Could you check a few things on this model? Use its own coordinates, in mm. Face numbers are marked on the shaded views. A direction names the side the tool comes from. Round coordinates to 2 decimals unless told otherwise and drop trailing zeros. Order: outer loops, then holes, each group sorted by start corner. A loop starts at its lowest first (then second) coordinate and runs counter-clockwise, first axis right, second up. Notation, with made-up numbers: M -23,-38.75 L -11,-38.75 A6 cw -11,-34.75 Z; hole C 41.25,-35 d5. An arc over 180 degrees is marked long. Write each question's results on one line, items separated by ' | '. Start each with the question number.
1. Suppose I cut it at C-C on x = -1. Write out the boundary of the cut face in (y, z), and give its area (4 significant figures).
2. Please list where these lines run through material, in increasing order: L1, parallel to X at y = 40.5, z = 5; L2, parallel to Y at x = 12.5, z = 1.4; L3, parallel to X at y = 30, z = 9.5.
3. Suppose I cut it at A-A on z = 13.5. Write out the boundary of the cut face in (x, y), and give its area (3 significant figures).
4. We'd pull the mould along X, two halves only. Please class the marked faces 1, 2 and 3: released by +X, released by -X, zero draft, split by the parting line, or undercut.
5. Suppose I cut it at B-B on y = 44. Write out the boundary of the cut face in (x, z).
6. I'm going to push flat-ended pins straight in: pin 1 (3 mm diameter, centred on y = 47.5, z = 3, fed in from -X); pin 2 (8 mm diameter, centred on x = 1, z = 5.5, fed in from +Y); pin 3 (1.8 mm diameter, centred on x = 12.5, y = 1.5, fed in from +Z); pin 4 (1.5 mm diameter, centred on x = 22, y = 0, fed in from +Z). Where does each tip first touch, or does it pass through?
7. For the marked faces 4, 5, 6, 7 and 8, which set-ups out of +Z, -Z, +X, -X, +Y, -Y let a thin tool reach every point of the face, with its end or its side?
8. Suppose I cut it at D-D on y = 22.5. Write out the boundary of the cut face in (x, z).
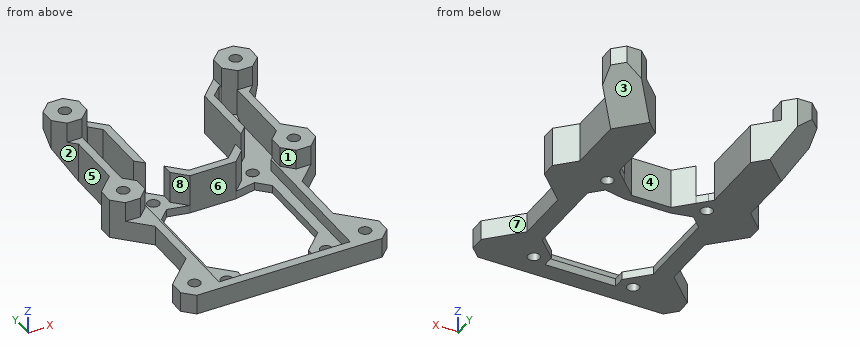
from build123d import *

# Parameters (mm, degrees)
SKETCH5_R           = 1.5
BOSS_EXTRUDE1_DEPTH = 2
SKETCH9_R           = 1.5
BOSS_EXTRUDE3_DEPTH = 3
SKETCH10_R          = 1.5
BOSS_EXTRUDE4_DEPTH = 5
BOSS_EXTRUDE5_DEPTH = 5.1
SKETCH13_R          = 1.5
CUT_EXTRUDE1_DEPTH  = 4.5
CUT_EXTRUDE2_DEPTH  = 7.5
CUT_EXTRUDE3_DEPTH  = 7.5
CHAMFER1_SIZE       = 1
CHAMFER1_SIZE2      = 1.191753593


with BuildPart() as part:
    # Sketch5 → Boss-Extrude1 (new body)
    with BuildSketch(Plane.XY):
        Polygon((19.636038969, -4.5), (-19.636038969, -4.5), (-23.363961031, -4.5), (-26, -1.863961031), (-26, 1.863961031), (-23.363961031, 4.5), (-18.5, 9.363961031), (-18.5, 23.636038969), (-23.363961031, 28.5), (-26, 31.136038969), (-26, 34.863961031), (-23.363961031, 37.5), (-21.5, 39.363961031), (-21.5, 53.636038969), (-23.363961031, 55.5), (-26, 58.136038969), (-26, 61.863961031), (-23.363961031, 64.5), (-19.636038969, 64.5), (-17, 61.863961031), (-12, 56.863961031), (-12, 40.029437252), (-11.050252532, 39.079689783), (-9, 37.029437252), (-4.970562748, 33), (4.970562748, 33), (9, 37.029437252), (11.050252532, 39.079689783), (12, 40.029437252), (12, 56.863961031), (17, 61.863961031), (19.636038969, 64.5), (23.363961031, 64.5), (26, 61.863961031), (26, 58.136038969), (23.363961031, 55.5), (21.5, 53.636038969), (21.5, 39.363961031), (23.363961031, 37.5), (26, 34.863961031), (26, 31.136038969), (23.363961031, 28.5), (18.5, 23.636038969), (18.5, 9.363961031), (23.363961031, 4.5), (26, 1.863961031), (26, -1.863961031), (23.363961031, -4.5), align=None)
        with Locations((-12.5, 35.579689783)):
            Circle(SKETCH5_R, mode=Mode.SUBTRACT)
        with Locations((-12.5, 1.5)):
            Circle(SKETCH5_R, mode=Mode.SUBTRACT)
        with Locations((12.5, 1.5)):
            Circle(SKETCH5_R, mode=Mode.SUBTRACT)
        with Locations((12.5, 35.579689783)):
            Circle(SKETCH5_R, mode=Mode.SUBTRACT)
        Polygon((-5.798989873, 31), (5.798989873, 31), (11.050252532, 32.079689783), (14, 29.129942315), (14, 8.121320344), (11, 5.121320344), (8.878679656, 3), (8.878679656, 0), (-8.878679656, 0), (-8.878679656, 3), (-11, 5.121320344), (-14, 8.121320344), (-14, 29.129942315), (-11.050252532, 32.079689783), align=None, mode=Mode.SUBTRACT)
    extrude(amount=BOSS_EXTRUDE1_DEPTH)

    # Sketch9 → Boss-Extrude3 (add)
    # profile 1 of 2: a face of its own
    with BuildSketch(Plane.XY.offset(2)):
        Polygon((19.636038969, -4.5), (-19.636038969, -4.5), (-23.363961031, -4.5), (-26, -1.863961031), (-26, 1.863961031), (-23.363961031, 4.5), (-18.5, 9.363961031), (-18.5, 23.636038969), (-23.363961031, 28.5), (-26, 31.136038969), (-26, 34.863961031), (-23.363961031, 37.5), (-21.5, 39.363961031), (-21.5, 53.636038969), (-23.363961031, 55.5), (-26, 58.136038969), (-26, 61.863961031), (-23.363961031, 64.5), (-19.636038969, 64.5), (-17, 61.863961031), (-12, 56.863961031), (-12, 40.029437252), (-14, 42.029437252), (-14, 56.035533906), (-16.550252532, 58.585786438), (-17, 58.136038969), (-19.5, 55.636038969), (-19.5, 37.363961031), (-17, 34.863961031), (-16.5, 34.363961031), (-16.5, -2.25), (16.5, -2.25), (16.5, 34.363961031), (17, 34.863961031), (19.5, 37.363961031), (19.5, 55.636038969), (17, 58.136038969), (16.550252532, 58.585786438), (14, 56.035533906), (14, 42.029437252), (12, 40.029437252), (12, 56.863961031), (17, 61.863961031), (19.636038969, 64.5), (23.363961031, 64.5), (26, 61.863961031), (26, 58.136038969), (23.363961031, 55.5), (21.5, 53.636038969), (21.5, 39.363961031), (23.363961031, 37.5), (26, 34.863961031), (26, 31.136038969), (23.363961031, 28.5), (18.5, 23.636038969), (18.5, 9.363961031), (23.363961031, 4.5), (26, 1.863961031), (26, -1.863961031), (23.363961031, -4.5), align=None)
        with Locations((-21.5, 0)):
            Circle(SKETCH9_R, mode=Mode.SUBTRACT)
        with Locations((-21.5, 33)):
            Circle(SKETCH9_R, mode=Mode.SUBTRACT)
        with Locations(Location((21.5, 33, 0), (0, 0, 180))):
            Circle(SKETCH9_R, mode=Mode.SUBTRACT)
        with Locations(Location((21.5, 0, 0), (0, 0, 180))):
            Circle(SKETCH9_R, mode=Mode.SUBTRACT)
    # profile 2 of 2: a face of its own
    with BuildSketch(Plane.XY.offset(2)):
        Polygon((4.970562748, 33), (-4.970562748, 33), (-9, 37.029437252), (-9, 34.201010127), (-5.798989873, 31), (5.798989873, 31), (9, 34.201010127), (9, 37.029437252), align=None)
    extrude(amount=BOSS_EXTRUDE3_DEPTH)

    # Sketch10 → Boss-Extrude4 (add)
    # profile 1 of 3: a face of its own
    with BuildSketch(Plane.XY.offset(5)):
        Polygon((-23.363961031, 28.5), (-19.636038969, 28.5), (-17, 31.136038969), (-17, 34.863961031), (-19.5, 37.363961031), (-19.5, 55.636038969), (-17, 58.136038969), (-16.550252532, 58.585786438), (-14, 56.035533906), (-14, 42.029437252), (-12, 40.029437252), (-12, 56.863961031), (-17, 61.863961031), (-19.636038969, 64.5), (-23.363961031, 64.5), (-26, 61.863961031), (-26, 58.136038969), (-23.363961031, 55.5), (-21.5, 53.636038969), (-21.5, 39.363961031), (-23.363961031, 37.5), (-26, 34.863961031), (-26, 31.136038969), align=None)
        with Locations((-21.5, 33)):
            Circle(SKETCH10_R, mode=Mode.SUBTRACT)
    # profile 2 of 3: a face of its own
    with BuildSketch(Plane.XY.offset(5)):
        Polygon((-9, 34.201010127), (-9, 37.029437252), (-4.970562748, 33), (4.970562748, 33), (9, 37.029437252), (9, 34.201010127), (5.798989873, 31), (-5.798989873, 31), align=None)
    # profile 3 of 3: a face of its own
    with BuildSketch(Plane.XY.offset(5)):
        Polygon((19.636038969, 28.5), (17, 31.136038969), (17, 34.863961031), (19.5, 37.363961031), (19.5, 55.636038969), (17, 58.136038969), (16.550252532, 58.585786438), (14, 56.035533906), (14, 42.029437252), (12, 40.029437252), (12, 56.863961031), (17, 61.863961031), (19.636038969, 64.5), (23.363961031, 64.5), (26, 61.863961031), (26, 58.136038969), (23.363961031, 55.5), (21.5, 53.636038969), (21.5, 39.363961031), (23.363961031, 37.5), (26, 34.863961031), (26, 31.136038969), (23.363961031, 28.5), align=None)
        with Locations(Location((21.5, 33, 0), (0, 0, 180))):
            Circle(SKETCH10_R, mode=Mode.SUBTRACT)
    extrude(amount=BOSS_EXTRUDE4_DEPTH)

    # Sketch12 → Boss-Extrude5 (add)
    with BuildSketch(Plane.XY.offset(10)):
        Polygon((-26, 58.136038969), (-23.363961031, 55.5), (-19.636038969, 55.5), (-17, 58.136038969), (-17, 61.863961031), (-19.636038969, 64.5), (-23.363961031, 64.5), (-26, 61.863961031), align=None)
        Polygon((17, 58.136038969), (17, 61.863961031), (19.636038969, 64.5), (23.363961031, 64.5), (26, 61.863961031), (26, 58.136038969), (23.363961031, 55.5), (19.636038969, 55.5), align=None)
    extrude(amount=BOSS_EXTRUDE5_DEPTH)

    # Sketch13 → Cut-Extrude1 (cut)
    with BuildSketch(Plane.XY.offset(15.1)):
        with Locations((-21.5, 60)):
            Circle(SKETCH13_R)
        with Locations(Location((21.5, 60, 0), (0, 0, 180))):
            Circle(SKETCH13_R)
    extrude(amount=-CUT_EXTRUDE1_DEPTH, mode=Mode.SUBTRACT)

    # Sketch15 → Cut-Extrude2 (cut, symmetric)
    with BuildSketch(Plane(origin=(19.25, 19.25, 0), x_dir=(0, 0, -1), z_dir=(0.7071067811865485, 0.7071067811865467, 0))):
        Polygon((0, 53.129202667), (-15.320888862, 65.98495486), (-8.893012766, 73.645399292), (6.427876097, 60.789647098), align=None)
    extrude(amount=CUT_EXTRUDE2_DEPTH, both=True, mode=Mode.SUBTRACT)

    # Sketch16 → Cut-Extrude3 (cut, symmetric)
    with BuildSketch(Plane(origin=(-19.25, 19.25, 0), x_dir=(0.7071067811865477, 0.7071067811865474, 0), z_dir=(-0.7071067811865474, 0.7071067811865477, 0))):
        Polygon((53.129202667, 0), (65.98495486, -15.320888862), (73.645399292, -8.893012766), (60.789647098, 6.427876097), align=None)
    extrude(amount=CUT_EXTRUDE3_DEPTH, both=True, mode=Mode.SUBTRACT)

    # Chamfer1
    chamfer1_edges = [part.edges().sort_by_distance(p)[0] for p in [
        (18.025126266, 57.110912703, 2),
        (-18.025126266, 57.110912703, 2),
    ]]
    chamfer1_side = [part.faces().sort_by_distance(p)[0] for p in [
        (-13.510979105, 40.518458147, 2),
    ]]
    chamfer(chamfer1_edges, length=CHAMFER1_SIZE, length2=CHAMFER1_SIZE2, reference=chamfer1_side[0])


solid = part.part
Filled sheet:
1) outline: M -4.5,0 L 0,0 L 0,2 L -2.25,2 L -2.25,5 L -4.5,5 Z; M 31,0 L 33,0 L 33,10 L 31,10 Z | area: 35.75 mm^2
2) L1: x = -21.5 to -19.5, -12.47 to -12, 12 to 12.47, 19.5 to 21.5 | L2: y = -4.5 to 0, 3 to 6.62, 30.63 to 34.08, 37.08 to 57.36 | L3: x = -24.86 to -18.14, 18.14 to 24.86
3) outline: M -26,58.14 L -23.36,55.5 L -19.64,55.5 L -17,58.14 L -17,61.86 L -19.64,64.5 L -23.36,64.5 L -26,61.86 Z; M 17,58.14 L 19.64,55.5 L 23.36,55.5 L 26,58.14 L 26,61.86 L 23.36,64.5 L 19.64,64.5 L 17,61.86 Z; hole C -21.5,60 d3; hole C 21.5,60 d3 | area: 120 mm^2
4) face 1: undercut | face 2: released by -X | face 3: released by +X
5) outline: M -21.5,0 L -12,0 L -12,10 L -14,10 L -14,2 L -19.5,2 L -19.5,10 L -21.5,10 Z; M 12,0 L 21.5,0 L 21.5,10 L 19.5,10 L 19.5,2 L 14,2 L 14,10 L 12,10 Z
6) pin 1: stops at x = -21.5 | pin 2: stops at y = 33.03 | pin 3: passes through | pin 4: stops at z = 2
7) face 4: +Z, -Z, +Y | face 5: +Z, -Z, -X | face 6: +Z, -Z | face 7: +Z, -Z, +X | face 8: +Z
8) outline: M -18.5,0 L -14,0 L -14,2 L -16.5,2 L -16.5,5 L -18.5,5 Z; M 14,0 L 18.5,0 L 18.5,5 L 16.5,5 L 16.5,2 L 14,2 Z
